The listing builds one solid part. Answer for the finished solid, in the listing's coordinates (mm). Give positions to 0.01 mm unless a question says otherwise; leave off trailing zeros. Order: outer loops, then holes, each group sorted by start corner. A loop starts at its lowest first (then second) coordinate and runs counter-clockwise, first axis right, second up. Notation, with made-up numbers: (-19, 10.5) - (34, 10.5) arc R20 cw to (34, 29.5) - close; hole circle Ø3 at (-37.75, 31). An arc over 180 degrees is marked (long way). Use CSV: the item, a comma, the result in double quotes.
```python
from build123d import *

# Parameters (mm, degrees)
F0_W     = 863.6
F0_H     = 76.2
F1_DEPTH = 9.525
F0_W_2   = 876.3
F0_H_2   = 88.9
F2_DEPTH = 3.175
F3_R     = 2.54


with BuildPart() as f1:
    # F0 (on Front) → F1 (new body)
    with BuildSketch(Plane.XZ):
        Rectangle(F0_W, F0_H)
    extrude(amount=F1_DEPTH)

    # F0 (on Front) → F2 (join)
    with BuildSketch(Plane.XZ):
        Rectangle(F0_W_2, F0_H_2)
        Rectangle(F0_W, F0_H, mode=Mode.SUBTRACT)
    extrude(amount=F2_DEPTH)

    # F3
    f3_edges = [f1.edges().sort_by_distance(p)[0] for p in [
        (431.8, -9.525, 0),
        (0, -9.525, 38.1),
        (-431.8, -9.525, 0),
        (0, -9.525, -38.1),
        (-438.15, -3.175, 0),
        (0, -3.175, -44.45),
        (438.15, -3.175, 0),
        (0, -3.175, 44.45),
        (-431.8, -3.175, 0),
        (0, -3.175, 38.1),
        (431.8, -3.175, 0),
        (0, -3.175, -38.1),
    ]]
    fillet(f3_edges, radius=F3_R)


solid = f1.part
```
Item 1: Find the intervals of material crossed by line 1 along X through (y, z) = (-6.5, -23.5); line 2 along Z through (x, y) = (-391, -5.5); line 3 along X through (y, z) = (-1.5, -31.5), in increasing order.
Taken from the geometry:
line 1,"-431.8 to 431.8"
line 2,"-38.11 to 38.11"
line 3,"-438 to 438"
Item 2: The part is cut by section A-A (x = 69.5). Give the vertices of the cut face in (y, z) (3 decimals), and give its area (3 significant figures).
Taken from the geometry:
outline,"(-9.525, -35.56) arc R2.54 ccw to (-6.985, -38.1) - (-5.715, -38.1) arc R2.54 cw to (-3.175, -40.64) - (-3.175, -41.91) arc R2.54 ccw to (-0.635, -44.45) - (0, -44.45) - (0, 44.45) - (-0.635, 44.45) arc R2.54 ccw to (-3.175, 41.91) - (-3.175, 40.64) arc R2.54 cw to (-5.715, 38.1) - (-6.985, 38.1) arc R2.54 ccw to (-9.525, 35.56) - close"
area,"763 mm^2"
Item 3: Each of these flat-tipped pins is pushed along its axis until it touches: pin 1 (5 mm diameter, centred on x = 229.5, y = -8, fed in from +Z); pin 2 (0.6 mm diameter, centred on y = -6, z = -1.5, fed in from -X); pin 3 (0.6 mm diameter, centred on y = -6.5, z = 0.5, fed in from +X). Where does it stop, or does it pass through?
Taken from the geometry:
pin 1,"z = 38.11"
pin 2,"x = -431.8"
pin 3,"x = 431.8"
